Design review of the part built by this model. Coordinates are the model's own, in mm. A direction names the side the tool comes from. Coordinates: 2 decimals unless noted, no trailing zeros. Loops run counter-clockwise (first coordinate to the right, second up) from the corner with the lowest first, then second, coordinate; pieces in that order, holes last. Notation, with made-up numbers: (63.5, -39.75) -> (69.5, -39.75) arc R26 cw to (69.5, -21.75) -> close; hole circle Ø2 at (89.5, -16). An arc over 180 degrees is marked (long way). Answer in a Markdown table with one row per item.
```python
from build123d import *

# Parameters (mm, degrees)
BOSS_EXTRUDE1_DEPTH        = 39.878
F_10_32_TAPPED_HOLE1_D     = 4.0386
F_10_32_TAPPED_HOLE1_DEPTH = 39.878
F_6_32_TAPPED_HOLE1_D      = 2.7051
F_6_32_TAPPED_HOLE1_DEPTH  = 6.35
CUT_EXTRUDE1_REACH         = 12.319
SKETCH10_R                 = 3.96875
F_4_40_TAPPED_HOLE1_D      = 2.2606
F_4_40_TAPPED_HOLE1_DEPTH  = 6.35
F_4_40_TAPPED_HOLE1_TIP    = 0.679152758


with BuildPart() as part:
    # Sketch1 → Boss-Extrude1 (new body)
    with BuildSketch(Plane(origin=(0, 0, 0), x_dir=(1, 0, 0), z_dir=(0, 1, 0))):
        Polygon((0, 0), (-3.96875, 0), (-3.96875, 9.525), (6.35, 9.525), (6.35, -10.31875), (0, -10.31875), align=None)
    extrude(amount=BOSS_EXTRUDE1_DEPTH)

    # #10-32 Tapped Hole1
    with Locations(Plane(origin=(0, 39.878, 0), x_dir=(1, 0, 0), z_dir=(0, 1, 0))):
        with Locations((1.11125, 4.7625)):
            Hole(F_10_32_TAPPED_HOLE1_D / 2, depth=F_10_32_TAPPED_HOLE1_DEPTH)

    # #6-32 Tapped Hole1
    with Locations(Plane.ZY):
        with Locations((5.159375, 13.97254)):
            Hole(F_6_32_TAPPED_HOLE1_D / 2, depth=F_6_32_TAPPED_HOLE1_DEPTH)

    # Sketch10 → Cut-Extrude1 (cut, up to next)
    with BuildSketch(Plane(origin=(6.35, 0, 0), x_dir=(0, 0, -1), z_dir=(1, 0, 0)), mode=Mode.PRIVATE) as cut_extrude1_sk1:
        with Locations((-5.159375, 24.47254)):
            Circle(SKETCH10_R)
    cut_extrude1_tool1 = extrude(cut_extrude1_sk1.sketch, amount=-CUT_EXTRUDE1_REACH, mode=Mode.PRIVATE) & part.part
    add(cut_extrude1_tool1.solids().sort_by_distance((6.35, 24.47254, 5.159375))[0], mode=Mode.SUBTRACT)

    # #4-40 Tapped Hole1
    with Locations(Plane(origin=(0, 39.878, 0), x_dir=(1, 0, 0), z_dir=(0, 1, 0))):
        with Locations((3.14325, -4.7625)):
            Hole(F_4_40_TAPPED_HOLE1_D / 2, depth=F_4_40_TAPPED_HOLE1_DEPTH)
            with Locations((0, 0, -(F_4_40_TAPPED_HOLE1_DEPTH + F_4_40_TAPPED_HOLE1_TIP / 2))):  # 118° drill point
                Cone(0, F_4_40_TAPPED_HOLE1_D / 2, F_4_40_TAPPED_HOLE1_TIP, mode=Mode.SUBTRACT)


solid = part.part
```
(1) Draft analysis for pull direction Y (two halves, no side actions). For faces 4 (the cylindrical face through (3.22, 20.6, 6.02)), 5 (the flat face through (2, 39.878, 0)), 6 (the flat face through (1, 20, -9.525)), 7 (the cylindrical face through (3.22, 15.11, 4.43)), state which applies: pulls with the +Y half, pulls with the -Y half, needs draft (parallel to the pull), parting line crosses it, or undercut.
Evaluation:
| item | result |
|---|---|
| face 4 | undercut |
| face 5 | pulls with the +Y half |
| face 6 | needs draft |
| face 7 | undercut |
(2) Take a section at B-B on x = 1.5. Give the boundary of the cut face in (y, z) (1 decimal), and give its area (3 significant figures).
Evaluation:
| item | result |
|---|---|
| outline | (0, -9.5) -> (39.9, -9.5) -> (39.9, -6.7) -> (0, -6.7) -> close; (0, -2.8) -> (39.9, -2.8) -> (39.9, 10.3) -> (0, 10.3) -> close; hole circle Ø2.7 at (14, 5.2); hole circle Ø7.9 at (24.5, 5.2) |
| area | 578 mm² |
(3) Tool access review of faces 1 (the cylindrical face through (4.272, 36.659, 4.713)), 2 (the flat face through (2, 0, 0)), 3 (the flat face through (-2, 20, 0)): name each direction out of +Z, -Z, +X, -X, +Y, -Y from which nothing blocks a thin tool from reaching the whole face with its end or side.
Evaluation:
| item | result |
|---|---|
| face 1 | +Y |
| face 2 | +Z, -Z, +X, -X, -Y |
| face 3 | +Z, -X, +Y, -Y |
(4) Take a section at A-A on y = 21. Count the separate pieces of the cut face and the enclosed holes in it, and give its area (3 significant figures).
Evaluation:
| item | result |
|---|---|
| separate pieces | 2 |
| enclosed holes | 1 |
| area | 127 mm² |
(5) For pin 1 (2 mm diameter, centred on x = -1.5, y = 20, fed in from +Z), flat-tipped, find the tip position at first contact; note if it passes through.
Evaluation:
| item | result |
|---|---|
| pin 1 | stops at z = 0 |
(6) To check wall thickness, follow probe 1 along Z at (x, y) = (2.75, 37) (3 decimals); probe 2 along Z at (x, y) = (-2.75, 32) (3 decimals); probe 3 along X at (y, z) = (7, 9.25). State the ranges of each line that lie inside material, in increasing order.
Evaluation:
| item | result |
|---|---|
| probe 1 | z = -9.525 to -5.942, -3.583 to 3.703, 5.822 to 10.319 |
| probe 2 | z = -9.525 to 0 |
| probe 3 | x = 0 to 6.35 |
